The model under review builds one solid part; all positions refer to its coordinate system, in mm. Face numbers are marked on the shaded views. Give positions to 0.01 mm unless a question says otherwise; leave off trailing zeros. Order: outer loops, then holes, each group sorted by start corner. A loop starts at its lowest first (then second) coordinate and runs counter-clockwise, first axis right, second up. Notation, with made-up numbers: (41.5, 83.25) - (65.5, 83.25) arc R21 cw to (65.5, 108.25) - close; hole circle Ø5 at (67.25, 70). An arc over 180 degrees is marked (long way). Answer as CSV lines item,"result". Start each with the question number.
from build123d import *

# Parameters (mm, degrees)
BASE_R_VOLUTION_ANGLE   = 358
ENL_V_MAT_EXTRU_3_DEPTH = 19.227726134


with BuildPart() as part:
    # Esquisse1 → Base-Révolution (revolve)
    with BuildSketch(Plane.XY):
        with BuildLine():
            Line((0, 7), (10, 7))
            ThreePointArc((10, 7), (10.353553391, 7.146446609), (10.5, 7.5))
            Line((10.5, 7.5), (10.5, 10))
            Line((10.5, 10), (11.5, 10))
            Line((11.5, 10), (11.5, 7.5))
            ThreePointArc((11.5, 7.5), (11.060660172, 6.439339828), (10, 6))
            Line((10, 6), (0, 6))
            Line((0, 6), (0, 7))
        make_face()
    revolve(axis=Axis((0, 0, 0), (1, 0, 0)), revolution_arc=BASE_R_VOLUTION_ANGLE)

    # Esquisse2 → Enlèv. mat.-Extru.3 (cut, through all)
    with BuildSketch(Plane(origin=(0, 0, 0), x_dir=(0, 0, -1), z_dir=(1, 0, 0))):
        Polygon((0.244296477, 6.995735789), (2.079990656, 9.933460569), (0.348994967, 9.99390827), (0, 10), (-1.732050808, 10), (0, 7), align=None)
    extrude(amount=ENL_V_MAT_EXTRU_3_DEPTH, mode=Mode.SUBTRACT)


solid = part.part
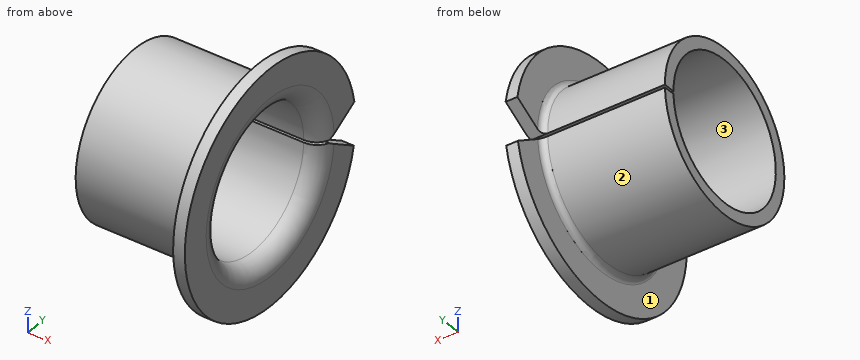
Item 1: Clearance check with flat-ended pins moving along their axes: pin 1 (4 mm diameter, centred on x = 6, z = 2, fed in from +Y); pin 2 (4 mm diameter, centred on x = 9, y = -4, fed in from -Z) (3 decimals); pin 3 (1.5 mm diameter, centred on x = 9.5, z = 4.5, fed in from +Y). State where each tip first meets the part, or that it passes through.
Item 2: Mouldability with a two-part tool opening along Y and no side actions: class the marked faces 1, 2 and 3 as released by +Y, released by -Y, zero draft, split by the parting line, or undercut.
Item 3: Take a section at A-A on y = 0. Write out the cut boundary in (x, z).
Item 4: Take a section at C-C on x = 6.5. Write out the cut boundary in (y, z).
Item 5: For line 1 along Z through (x, y) = (7.25, 0); line 2 along Y through (x, z) = (5.5, -4.25); line 3 along Z through (x, y) = (6.25, 4), list the stretches that pass through material, from the lowest coordinate up.
Item 6: Take a section at B-B on y = 8. Write out the cut boundary in (x, z).
Data:
1,pin 1,"stops at y = 7"
1,pin 2,"stops at z = -9.635"
1,pin 3,"stops at y = 5.91"
2,face 1,"zero draft"
2,face 2,"split by the parting line"
2,face 3,"undercut"
3,outline,"(0, -7) - (10, -7) arc R0.5 cw to (10.5, -7.5) - (10.5, -10) - (11.5, -10) - (11.5, -7.5) arc R1.5 ccw to (10, -6) - (0, -6) - close; (0, 6) - (10, 6) arc R1.5 ccw to (11.5, 7.5) - (11.5, 10) - (10.5, 10) - (10.5, 7.5) arc R0.5 cw to (10, 7) - (0, 7) - close"
4,outline,"(6, -0.21) arc R6 cw (long way) to (6, 0) - (7, 0) arc R7 ccw (long way) to (7, -0.24) - close"
5,line 1,"z = -7 to -6, 6 to 7"
5,line 2,"y = -5.56 to -4.24, 4.24 to 5.56"
5,line 3,"z = -5.74 to -4.47, 4.47 to 5.74"
6,outline,"(10.5, -6) - (11.5, -6) - (11.5, -0.87) - (10.5, -0.87) - close; (10.5, 0.58) - (11.5, 0.58) - (11.5, 6) - (10.5, 6) - close"
